from build123d import *

# Parameters (mm, degrees)
SKETCH1_R             = 3.38
SKETCH1_W             = 23
SKETCH1_H             = 23
SKETCH1_R_2           = 1.13
SKETCH1_R_3           = 3.175
BOSS_EXTRUDE1_DEPTH   = 2.54
F_4_40_TAPPED_HOLE1_D = 2.2606
FILLET1_R             = 10


with BuildPart() as part:
    # Sketch1 → Boss-Extrude1 (new body)
    with BuildSketch(Plane.XY):
        with BuildLine():
            Line((101.231699996, -8e-08), (41.425999995, -8e-08))
            Line((41.425999995, -8e-08), (41.425999995, -13.716000085))
            Line((41.425999995, -13.716000085), (20.065999995, -13.716000085))
            Line((20.065999995, -13.716000085), (13.715999995, -20.066000085))
            Line((13.715999995, -20.066000085), (13.715999995, -192.786000085))
            Line((13.715999995, -192.786000085), (20.065999995, -199.136000085))
            Line((20.065999995, -199.136000085), (41.425999995, -199.136000085))
            Line((41.425999995, -199.136000085), (41.425999995, -212.852000091))
            Line((41.425999995, -212.852000091), (101.231699997, -212.852000091))
            Line((101.231699997, -212.852000091), (101.231699997, -208.02600019))
            ThreePointArc((101.231699996, -208.02600019), (106.425999995, -202.83170019), (111.620299995, -208.02600019))
            Line((111.620299996, -208.02600019), (111.620299996, -212.852000091))
            Line((111.620299996, -212.852000091), (195.854149957, -212.852000091))
            Line((195.854149957, -212.852000091), (212.851999956, -195.854150092))
            Line((212.851999956, -195.854150092), (212.851999956, -111.620300137))
            Line((212.851999956, -111.620300137), (208.026000047, -111.620300137))
            ThreePointArc((208.026000047, -111.620300137), (202.831700048, -106.426000137), (208.026000047, -101.231700138))
            Line((208.026000047, -101.231700138), (212.851999956, -101.231700138))
            Line((212.851999956, -101.231700138), (212.851999956, -16.997850079))
            Line((212.851999956, -16.997850079), (195.854149957, -8e-08))
            Line((195.854149957, -8e-08), (111.620299995, -8e-08))
            Line((111.620299995, -8e-08), (111.620299995, -4.826000085))
            ThreePointArc((111.620299994, -4.826000085), (106.425999995, -10.020300084), (101.231699996, -4.826000085))
            Line((101.231699996, -4.826000085), (101.231699996, -8e-08))
        make_face()
        with Locations((55.625999995, -208.02600019)):
            Circle(SKETCH1_R, mode=Mode.SUBTRACT)
        with Locations((81.025999995, -208.02600019)):
            Circle(SKETCH1_R, mode=Mode.SUBTRACT)
        with Locations((131.825999995, -208.02600019)):
            Circle(SKETCH1_R, mode=Mode.SUBTRACT)
        with Locations((157.225999995, -208.02600019)):
            Circle(SKETCH1_R, mode=Mode.SUBTRACT)
        with Locations((182.625999995, -208.02600019)):
            Circle(SKETCH1_R, mode=Mode.SUBTRACT)
        with Locations((208.026000047, -182.626000137)):
            Circle(SKETCH1_R, mode=Mode.SUBTRACT)
        with Locations((208.026000047, -157.226000137)):
            Circle(SKETCH1_R, mode=Mode.SUBTRACT)
        with Locations((208.026000047, -131.826000137)):
            Circle(SKETCH1_R, mode=Mode.SUBTRACT)
        with Locations((55.625999995, -4.826000085)):
            Circle(SKETCH1_R, mode=Mode.SUBTRACT)
        with Locations((81.025999995, -4.826000085)):
            Circle(SKETCH1_R, mode=Mode.SUBTRACT)
        with Locations((208.026000047, -81.026000137)):
            Circle(SKETCH1_R, mode=Mode.SUBTRACT)
        with Locations((208.026000047, -55.626000137)):
            Circle(SKETCH1_R, mode=Mode.SUBTRACT)
        with Locations((131.825999995, -4.826000085)):
            Circle(SKETCH1_R, mode=Mode.SUBTRACT)
        with Locations((157.225999995, -4.826000085)):
            Circle(SKETCH1_R, mode=Mode.SUBTRACT)
        with Locations((208.026000047, -30.226000137)):
            Circle(SKETCH1_R, mode=Mode.SUBTRACT)
        with Locations((182.625999995, -4.826000085)):
            Circle(SKETCH1_R, mode=Mode.SUBTRACT)
        with Locations((106.426000003, -65.34289)):
            Rectangle(SKETCH1_W, SKETCH1_H, mode=Mode.SUBTRACT)
        with Locations((119.876000003, -51.89289)):
            Circle(SKETCH1_R_2, mode=Mode.SUBTRACT)
        with Locations((92.976000003, -78.79289)):
            Circle(SKETCH1_R_2, mode=Mode.SUBTRACT)
        with Locations((45, -40)):
            Circle(SKETCH1_R_3, mode=Mode.SUBTRACT)
        with Locations((92.976000003, -51.89289)):
            Circle(SKETCH1_R_2, mode=Mode.SUBTRACT)
        with Locations((119.876000003, -78.79289)):
            Circle(SKETCH1_R_2, mode=Mode.SUBTRACT)
    extrude(amount=BOSS_EXTRUDE1_DEPTH)

    # #4-40 Tapped Hole1 (through all)
    with Locations(Plane(origin=(92.976000003, -51.89289, 2.54), x_dir=(1, 0, 0), z_dir=(0, 0, 1))):
        with Locations((0, 0), (26.9, 0), (26.9, -26.9), (0, -26.9)):
            Hole(F_4_40_TAPPED_HOLE1_D / 2)

    # Fillet1
    fillet1_edges = [part.edges().sort_by_distance(p)[0] for p in [
        (101.231699997, -212.852000091, 1.27),
        (111.620299996, -212.852000091, 1.27),
        (212.851999956, -111.620300137, 1.27),
        (212.851999956, -101.231700138, 1.27),
        (111.620299995, -8e-08, 1.27),
        (101.231699996, -8e-08, 1.27),
    ]]
    fillet(fillet1_edges, radius=FILLET1_R)


solid = part.part
Geometry check sheet. Reference: the model listing, model coordinates, mm. Round coordinates to 2 decimals unless told otherwise and drop trailing zeros. Loops run counter-clockwise (first coordinate to the right, second up) from the corner with the lowest first, then second, coordinate; pieces in that order, holes last.
Item 1: Cross-section at C-C on x = 183.5. Record the boundary of the cut face in (y, z).
Item 2: Cross-section at A-A on y = -40. Record the boundary of the cut face in (x, z) (3 decimals), then the cut area to 3 significant figures.
Item 3: Cross-section at B-B on x = 45. Record the boundary of the cut face in (y, z) (3 decimals), then the cut area to 3 significant figures.
Item 4: Gauge pin test, flat ends, axial feed: pin 1 (6 mm diameter, centred on x = 81.026, y = -4.826, fed in from -Z); pin 2 (1.3 mm diameter, centred on y = -7, z = 1.5, fed in from -X); pin 3 (0.8 mm diameter, centred on x = 29, z = 0.5, fed in from -Y); pin 4 (0.8 mm diameter, centred on x = 34, z = 1.5, fed in from +Y). Record the tip position at first contact, or that the pin passes through.
Item 5: Thickness scan on line 1 (X direction, y = -76, z = 0.3); line 2 (Y direction, x = 129.5, z = 1.35); line 3 (Y direction, x = 84, z = 1.5). Record the ranges inside material, lowest first.
Item 6: Mould release check, pull along Y, two halves, no side actions. Record for faces 1 (the cylindrical face through (160.45, -3.81, 1.25)), 2 (the flat face through (112, -105, 0)), 3 (the flat face through (16.935, -16.847, 1.252)), 4 (the flat face through (16.85, -195.92, 1.25)): pulls with the +Y half, pulls with the -Y half, needs draft (parallel to the pull), parting line crosses it, or undercut.
Item 7: Cross-section at D-D on z = 1.55. Count the separate pieces of the cut face and the enclosed holes in it, then the cut area to 3 significant figures.
Answer sheet:
1. outline: (-212.85, 0) - (-211.29, 0) - (-211.29, 2.54) - (-212.85, 2.54) - close; (-204.76, 0) - (-8.09, 0) - (-8.09, 2.54) - (-204.76, 2.54) - close; (-1.56, 0) - (0, 0) - (0, 2.54) - (-1.56, 2.54) - close
2. outline: (13.716, 0) - (41.825, 0) - (41.825, 2.54) - (13.716, 2.54) - close; (48.175, 0) - (212.852, 0) - (212.852, 2.54) - (48.175, 2.54) - close
2. area: 490 mm2
3. outline: (-212.852, 0) - (-43.175, 0) - (-43.175, 2.54) - (-212.852, 2.54) - close; (-36.825, 0) - (0, 0) - (0, 2.54) - (-36.825, 2.54) - close
3. area: 525 mm2
4. pin 1: passes through
4. pin 2: stops at x = 41.43
4. pin 3: stops at y = -199.14
4. pin 4: stops at y = -13.72
5. line 1: x = 13.72 to 94.93, 117.93 to 212.85
5. line 2: y = -212.85 to -210.48, -205.57 to -7.28, -2.37 to 0
5. line 3: y = -212.85 to -209.63, -206.42 to -6.43, -3.22 to 0
6. face 1: undercut
6. face 2: needs draft
6. face 3: pulls with the +Y half
6. face 4: pulls with the -Y half
7. separate pieces: 1
7. enclosed holes: 22
7. area: 39,800 mm2
